Could you check a few things on this model? Use its own coordinates, in mm. A direction names the side the tool comes from. Coordinates: 2 decimals unless noted, no trailing zeros. Order: outer loops, then holes, each group sorted by start corner. A loop starts at its lowest first (then second) coordinate and runs counter-clockwise, first axis right, second up. Notation, with made-up numbers: (9.5, 37.5) -> (36.5, 37.5) arc R34 cw to (36.5, 71.5) -> close; hole circle Ø2 at (68, 8). An arc over 180 degrees is marked (long way). Use a Markdown table: item, result. Add a question column.
1) Will these pins go through, and if not, where does the flat tip stop? pin 1 Ø9 at (y, z) = (-47.5, -63.7) entering from +X; pin 2 Ø8 at (x, z) = (48.5, -113) entering from +Y; pin 3 Ø2.5 at (x, y) = (4, -76.5) entering from +Z.
2) If we section it at A-A (z = -63.7): Write out the boundary of the cut face in (x, y).
3) Thinking about a two-plate mould opening in Z: for faces 1 (the cylindrical face through (11.4, -47.26, -58.15)), 2 (the flat face through (-2, 1, 125)), 3 (the cylindrical face through (11.4, 47.74, 107.85)), 4 (the flat face through (110, -1, 2)), which applies, +Z half, -Z half, draft (parallel to the pull), parting line (faces both ways), or undercut?
4) If I drill on L1, parallel to Y at x = 13, z = 102; L2, parallel to Y at x = 46.5, z = -63.7; L3, parallel to Z at x = -8, y = 47, over which ranges is the centre line in solid material (lowest first)? Write a range as [from, to].
5) If we section it at B-B (x = -10.5): Write out the boundary of the cut face in (y, z).
6) Which directions (+Z, -Z, +X, -X, +Y, -Y) give clear straight access to the entire face, cutting with the end or side of a thin tool? Please do faces 5 (the cylindrical face through (-15.62, -107.04, -3.47)), 6 (the flat face through (-90, 48, 102)), 7 (the flat face through (87, 1, -125)).
7) If we section it at D-D (z = 0): Write out the boundary of the cut face in (x, y), plus the area to 3 significant figures.
8) If we section it at C-C (y = -1.5): Write out the boundary of the cut face in (x, z), plus the area to 3 significant figures.
```python
from build123d import *

# Parameters (mm, degrees)
CROQUIS1_W              = 220
CROQUIS1_H              = 150
SALIENTE_EXTRUIR1_DEPTH = 125
CROQUIS2_R              = 16
SALIENTE_EXTRUIR2_DEPTH = 140
CROQUIS3_R              = 5.55625
CORTAR_EXTRUIR1_DEPTH   = 200
CROQUIS4_R              = 80
SALIENTE_EXTRUIR3_DEPTH = 270


with BuildPart() as part:
    # Croquis1 → Saliente-Extruir1 (new, symmetric)
    with BuildSketch(Plane.XY):
        Rectangle(CROQUIS1_W, CROQUIS1_H)
    extrude(amount=SALIENTE_EXTRUIR1_DEPTH, both=True)

    # Croquis2 → Saliente-Extruir2 (add, symmetric)
    with BuildSketch(Plane(origin=(0, 0, 0), x_dir=(1, 0, 0), z_dir=(0, 1, 0))):
        with Locations(Location((0, 0, 0), (0, 0, 270))):
            Circle(CROQUIS2_R)
    extrude(amount=SALIENTE_EXTRUIR2_DEPTH, both=True)

    # Croquis3 → Cortar-Extruir1 (cut)
    with BuildSketch(Plane(origin=(110, 0, 0), x_dir=(0, 0, -1), z_dir=(1, 0, 0))):
        with Locations((-102.3, 47.5)):
            Circle(CROQUIS3_R)
        with Locations((-102.3, -47.5)):
            Circle(CROQUIS3_R)
        with Locations((63.7, 47.5)):
            Circle(CROQUIS3_R)
        with Locations((63.7, -47.5)):
            Circle(CROQUIS3_R)
    extrude(amount=-CORTAR_EXTRUIR1_DEPTH, mode=Mode.SUBTRACT)

    # Croquis4 → Saliente-Extruir3 (add)
    with BuildSketch(Plane(origin=(0, 0, -125), x_dir=(-1, 0, 0), z_dir=(0, 0, -1))):
        with Locations(Location((0, 0, 0), (0, 0, 110.364134806))):
            Circle(CROQUIS4_R)
    extrude(amount=SALIENTE_EXTRUIR3_DEPTH)


solid = part.part
```
Answer sheet:
| question | item | result |
|---|---|---|
| 1 | pin 1 | x = -90 |
| 1 | pin 2 | y = 75 |
| 1 | pin 3 | z = 15.76 |
| 2 | outline | (-110, -75) -> (110, -75) -> (110, -53.06) -> (-90, -53.06) -> (-90, -41.94) -> (110, -41.94) -> (110, 41.94) -> (-90, 41.94) -> (-90, 53.06) -> (110, 53.06) -> (110, 75) -> (-110, 75) -> close |
| 3 | face 1 | undercut |
| 3 | face 2 | +Z half |
| 3 | face 3 | undercut |
| 3 | face 4 | draft |
| 4 | L1 | [-75, -53.05], [-41.95, 41.95], [53.05, 75] |
| 4 | L2 | [-75, -53.06], [-41.94, 41.94], [53.06, 75] |
| 4 | L3 | [-395, -69.23], [-58.17, 96.77], [107.83, 125] |
| 5 | outline | (-140, -12.07) -> (-75, -12.07) -> (-75, -125) -> (-79.31, -125) -> (-79.31, -395) -> (79.31, -395) -> (79.31, -125) -> (75, -125) -> (75, -12.07) -> (140, -12.07) -> (140, 12.07) -> (75, 12.07) -> (75, 125) -> (-75, 125) -> (-75, 12.07) -> (-140, 12.07) -> close; hole circle Ø11.11 at (-47.5, -63.7); hole circle Ø11.11 at (-47.5, 102.3); hole circle Ø11.11 at (47.5, -63.7); hole circle Ø11.11 at (47.5, 102.3) |
| 6 | face 5 | -Y |
| 6 | face 6 | +X |
| 6 | face 7 | -Z, +X |
| 7 | outline | (-110, -75) -> (-16, -75) -> (-16, -140) -> (16, -140) -> (16, -75) -> (110, -75) -> (110, 75) -> (16, 75) -> (16, 140) -> (-16, 140) -> (-16, 75) -> (-110, 75) -> close |
| 7 | area | 37,200 mm2 |
| 8 | outline | (-110, -125) -> (-79.99, -125) -> (-79.99, -395) -> (79.99, -395) -> (79.99, -125) -> (110, -125) -> (110, 125) -> (-110, 125) -> close |
| 8 | area | 98,200 mm2 |
